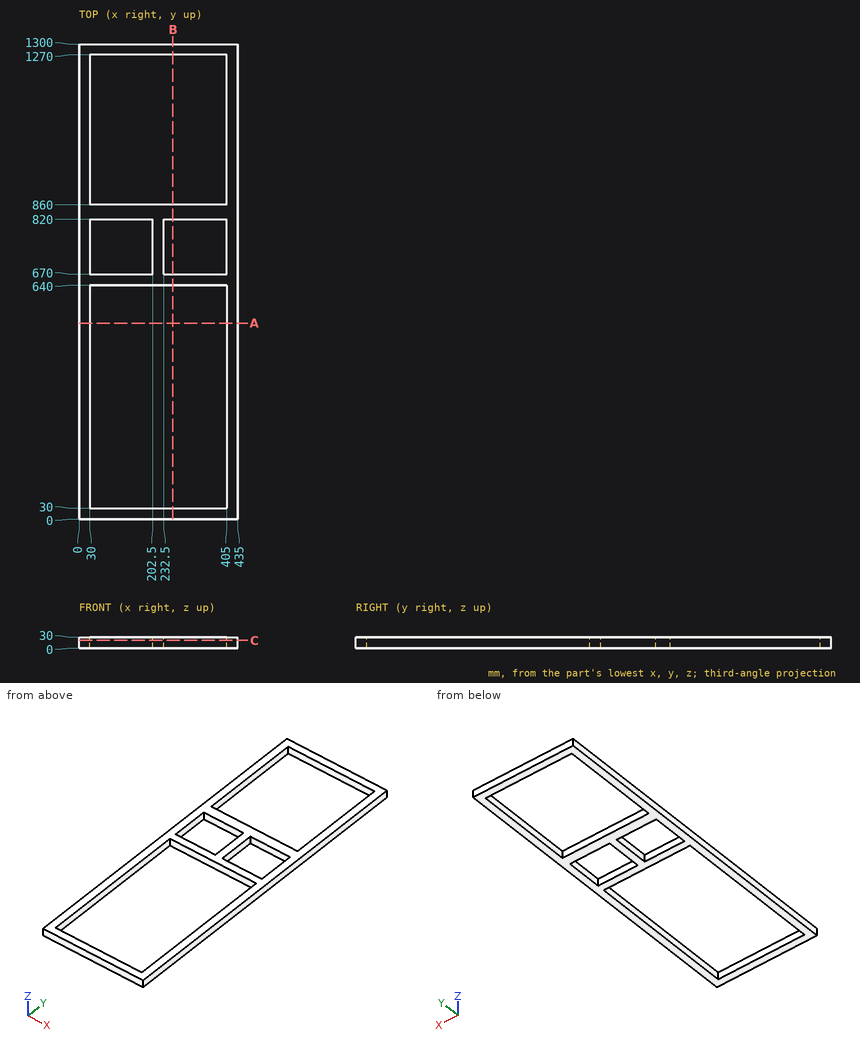
Input: dimensioned drawing with shaded views. Units: mm. Origin: part minimum x, y, z. Round coordinates to 2 decimals unless told otherwise and drop trailing zeros. Order: outer loops, then holes, each group sorted by start corner. A loop starts at its lowest first (then second) coordinate and runs counter-clockwise, first axis right, second up. Notation, with made-up numbers: (-11, -11.75) - (-3, -11.75) arc R25 ccw to (-3, 19.25) - close; hole circle Ø3 at (-2, 32). An arc over 180 degrees is marked (long way). Answer as a JSON object with one key per item and string values. Group by question number.
(1) Cut plane B-B (x = 257). Return loops of the section in (y, z).
(2) Cut plane A-A (y = 536). Return loops of the section in (x, z).
(3) Material intervals for probe 1 along Y at (x, z) = (374.5, 11.5); probe 2 along X at (y, z) = (401, 24); probe 3 along X at (y, z) = (798, 27.25), sorted ascending. Write a range as from..to.
(4) Cut plane C-C (z = 20.75). Return loops of the section in (x, y).
Here are the results:
{
 "1": {"outline": "(0, 0) - (30, 0) - (30, 30) - (0, 30) - close; (640, 0) - (670, 0) - (670, 30) - (640, 30) - close; (820, 0) - (860, 0) - (860, 30) - (820, 30) - close; (1270, 0) - (1300, 0) - (1300, 30) - (1270, 30) - close"},
 "2": {"outline": "(0, 0) - (30, 0) - (30, 30) - (0, 30) - close; (405, 0) - (435, 0) - (435, 30) - (405, 30) - close"},
 "3": {"probe 1": "y = 0..30, 640..670, 820..860, 1270..1300", "probe 2": "x = 0..30, 405..435", "probe 3": "x = 0..30, 202.5..232.5, 405..435"},
 "4": {"outline": "(0, 0) - (435, 0) - (435, 1300) - (0, 1300) - close; hole (30, 30) - (405, 30) - (405, 640) - (30, 640) - close; hole (30, 670) - (202.5, 670) - (202.5, 820) - (30, 820) - close; hole (30, 860) - (405, 860) - (405, 1270) - (30, 1270) - close; hole (232.5, 670) - (405, 670) - (405, 820) - (232.5, 820) - close"}
}
